Study the drawing (mm; zero at the part's minimum x, y, z) and answer. A direction names the side the tool comes from. Give positions to 0.01 mm unless a question says otherwise; leave off trailing zeros. Order: outer loops, then holes, each group sorted by start corner. A loop starts at its lowest first (then second) coordinate and runs counter-clockwise, first axis right, second up.
Item 1: Find the intervals of material crossed by line 1 along Z through (x, y) = (0.85, 3.8); line 2 along Y through (x, z) = (1.4, 2.25); line 3 along X through (y, z) = (2.25, 4.25), in increasing order.
Item 2: Given pin 1 Ø1.5 at (x, z) = (3, 3.5) entering from -Y; pin 2 Ø1.5 at (x, y) = (2, 1) entering from -Z; pin 3 Ø0.9 at (y, z) = (2.5, 5.5) entering from -X; pin 4 Ø0.9 at (y, z) = (2, 4.5) entering from +X, each flat-ended and moving along its own axis, determine where each tip first touches the part or whether it passes through.
Item 3: A cutting plane is placed at A-A (x = 2.4). Write down the section's boundary in (y, z).
Item 4: A cutting plane is placed at B-B (y = 1.65). Write down the section's boundary in (x, z), plus the area to 3 significant figures.
Item 5: The mould has two halves that part along Z. Classify the marked faces 4, 5, 6 and 7: +Z half, -Z half, draft (parallel to the pull), parting line (faces both ways), or undercut.
Item 6: Which of the six approach directions +Z, -Z, +X, -X, +Y, -Y give full straight-line access (tool end or side, diameter ignored) to the marked faces 1, 2 and 3?
Item 7: A cutting plane is placed at C-C (z = 1.5). Write down the section's boundary in (x, y), plus the area to 3 significant figures.
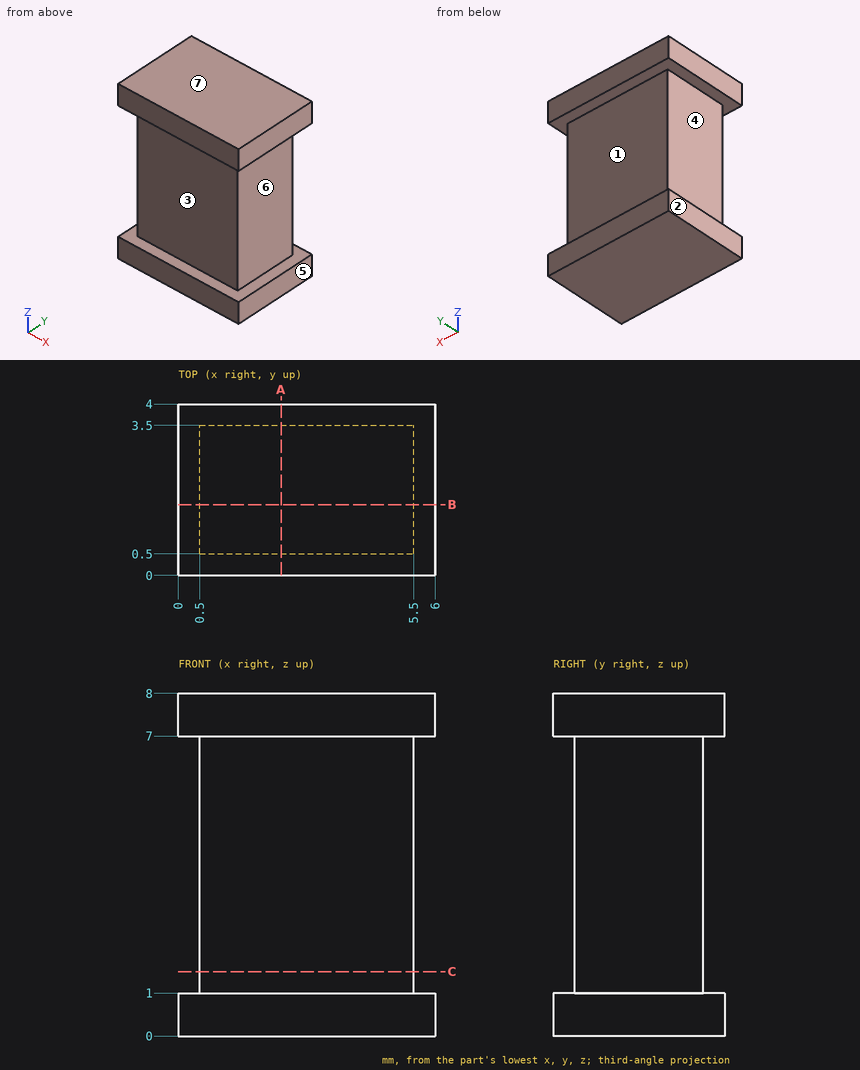
Response values:
1. line 1: z = 0 to 1, 7 to 8
1. line 2: y = 0.5 to 3.5
1. line 3: x = 0.5 to 5.5
2. pin 1: stops at y = 0.5
2. pin 2: stops at z = 0
2. pin 3: stops at x = 0.5
2. pin 4: stops at x = 5.5
3. outline: (0, 0) - (4, 0) - (4, 1) - (3.5, 1) - (3.5, 7) - (4, 7) - (4, 8) - (0, 8) - (0, 7) - (0.5, 7) - (0.5, 1) - (0, 1) - close
4. outline: (0, 0) - (6, 0) - (6, 1) - (5.5, 1) - (5.5, 7) - (6, 7) - (6, 8) - (0, 8) - (0, 7) - (0.5, 7) - (0.5, 1) - (0, 1) - close
4. area: 42.0 mm2
5. face 4: undercut
5. face 5: draft
5. face 6: undercut
5. face 7: +Z half
6. face 1: +X, -X, +Y
6. face 2: +Z, -Z, -X, +Y, -Y
6. face 3: +X, -X, -Y
7. outline: (0.5, 0.5) - (5.5, 0.5) - (5.5, 3.5) - (0.5, 3.5) - close
7. area: 15.0 mm2
